Input: part model. Units: mm. Frame: model coordinates. A direction names the side the tool comes from. Coordinates: 2 decimals unless noted, no trailing zeros. Write each loop counter-clockwise with the first axis right and the second up, starting at its lowest first coordinate (ties: lowest second). Pieces come first, ordered by that corner, then holes. Notation, with made-up numbers: (-30.5, -7) - (-21.5, -7) arc R22 cw to (-21.5, 10) - close; hole circle Ø11 at (-28.75, 41.25). An arc over 180 degrees is marked (long way). Put each result on its own line as item: value. Start each with the question number.
1. Access query for faces 1 (the flat face through (0.154, -59.263, -13.315)), 2 (the flat face through (-10, 13, -9)), 3 (the flat face through (11, -33, 0)), 4 (the flat face through (0, 0, 17)). Directions: +Z, -Z, +X, -X, +Y, -Y. A direction counts if a zero-diameter tool reaches every point of the face in a straight line with its end or side. Return the directions, or none.
2. Cut plane A-A, the plane x = 0. Return loops of the section in (y, z).
3. Cut plane B-B, the plane y = -46.5. Return loops of the section in (x, z).
4. Line query: line 1 (Y direction, x = 0, z = -0.75); line 2 (Y direction, x = 13, z = 18.5); line 3 (X direction, y = -63, z = -13). Output: solid intervals per line, ascending.
5. Pin query (flat end, axial travel): pin 1 (12 mm diameter, centred on x = 14.5, z = 2, fed in from -Y); pin 2 (1.5 mm diameter, centred on x = -3, z = -3.5, fed in from -Y); pin 3 (3 mm diameter, centred on x = -5.5, y = 6.5, fed in from +Z). Return the tip coordinate at first contact, or that it passes through.
6. Cut plane C-C, the plane z = -7.5. Return loops of the section in (x, y).
7. Cut plane D-D, the plane x = 9.5. Return loops of the section in (y, z), and give its area (3 significant figures).
8. Pull-direction query (Y, two-part tool) for faces 5 (the cylindrical face through (0, 47, 0)), 6 (the flat face through (17, -25, 0)), 7 (the cylindrical face through (-3.252, 10.357, 0.126)); classes: released by +Y, released by -Y, zero draft, split by the parting line, or undercut.
from build123d import *

# Parameters (mm, degrees)
BOSS_EXTRUDE2_DEPTH = 9
BOSS_EXTRUDE3_DEPTH = 22
BOSS_EXTRUDE5_START = -11
BOSS_EXTRUDE5_DEPTH = 22
SKETCH4_R           = 15
CUT_EXTRUDE1_DEPTH  = 44


with BuildPart() as part:
    # Sketch1 → Boss-Extrude2 (new body)
    with BuildSketch(Plane(origin=(0, 0, 0), x_dir=(0, 1, 0), z_dir=(0, 0, 1))):
        with BuildLine():
            Line((0, 22), (25, 22))
            ThreePointArc((25, 22), (47, 0), (25, -22))
            Line((25, -22), (0, -22))
            Line((0, -22), (0, 22))
        make_face()
    extrude(amount=BOSS_EXTRUDE2_DEPTH)

    # Sketch2 → Boss-Extrude3 (add, symmetric)
    with BuildSketch(Plane.YZ):
        Polygon((25, 0), (25, 9), (0, 9), (0, 25), (-25, 25), (-25, 0), (0, 0), align=None)
    extrude(amount=BOSS_EXTRUDE3_DEPTH, both=True)

    # Sketch3 → Boss-Extrude5 (add)
    with BuildSketch(Plane.YZ.offset(22).offset(BOSS_EXTRUDE5_START)):
        with BuildLine():
            Line((-25, 25), (-51, 25))
            ThreePointArc((-51, 25), (-59.593288161, 23.476699056), (-67.139363205, 19.092431886))
            ThreePointArc((-67.139363205, 19.092431886), (-68.101737646, 14.184187501), (-63.521788912, 12.173939479))
            Line((-63.521788912, 12.173939479), (-54.882285677, 14.488887394))
            ThreePointArc((-54.882285677, 14.488887394), (-41.868578565, 11.900300104), (-36, 0))
            Line((-36, 0), (-25, 0))
            Line((-25, 0), (-25, 25))
        make_face()
    extrude(amount=-BOSS_EXTRUDE5_DEPTH)

    # Mirror1: part across plane


with BuildPart() as part_1:
    add(part.part)
    add(part.part.mirror(Plane(origin=(0, 25, 0), x_dir=(1, 0, 0), z_dir=(0, 0, 1))))

    # Sketch4 → Cut-Extrude1 (cut)
    with BuildSketch(Plane.XY.offset(9)):
        with Locations((0, 25)):
            Circle(SKETCH4_R)
    extrude(amount=-CUT_EXTRUDE1_DEPTH, mode=Mode.SUBTRACT)


solid = part_1.part
Report:
1. face 1: +X, -X
1. face 2: -Z, +X, -X, +Y
1. face 3: +Z, -Z, +X, -Y
1. face 4: +Z, +X, -X, +Y
2. outline: (-67.14, -19.09) arc R25 ccw to (-51, -25) - (0, -25) - (0, -9) - (10, -9) - (10, 9) - (0, 9) - (0, 25) - (-51, 25) arc R25 ccw to (-67.14, 19.09) arc R4 ccw to (-63.52, 12.17) - (-54.88, 14.49) arc R15 cw (long way) to (-54.88, -14.49) - (-63.52, -12.17) arc R4 ccw to start; (40, -9) - (47, -9) - (47, 9) - (40, 9) - close
3. outline: (-11, -25) - (11, -25) - (11, -14.31) - (-11, -14.31) - close; (-11, 14.31) - (11, 14.31) - (11, 25) - (-11, 25) - close
4. line 1: y = -36.02 to 10, 40 to 47
4. line 2: y = -25 to 0
4. line 3: x = -11 to 11
5. pin 1: stops at y = -37.67
5. pin 2: stops at y = -36.61
5. pin 3: stops at z = 9
6. outline: (-22, -25) - (-11, -25) - (-11, -38.01) - (11, -38.01) - (11, -25) - (22, -25) - (22, 25) arc R22 ccw to (-22, 25) - close; hole circle Ø30 at (0, 25)
7. outline: (-67.14, -19.09) arc R25 ccw to (-51, -25) - (0, -25) - (0, -9) - (13.39, -9) - (13.39, 9) - (0, 9) - (0, 25) - (-51, 25) arc R25 ccw to (-67.14, 19.09) arc R4 ccw to (-63.52, 12.17) - (-54.88, 14.49) arc R15 cw (long way) to (-54.88, -14.49) - (-63.52, -12.17) arc R4 ccw to start; (36.61, -9) - (44.84, -9) - (44.84, 9) - (36.61, 9) - close
7. area: 2,910 mm^2
8. face 5: released by +Y
8. face 6: released by -Y
8. face 7: undercut
